```python
from build123d import *

# Parameters (mm, degrees)
EXTRUDE_1_DEPTH     = 33
CUT_EXTRUDE_1_REACH = 63.465
SKETCH_2_R          = 1.5
CUT_EXTRUDE_2_REACH = 63.952
SKETCH_3_R          = 2


with BuildPart() as part:
    # 草图1 → 凸台-拉伸1 (new body)
    with BuildSketch(Plane(origin=(0, 0, 0), x_dir=(1, 0, 0), z_dir=(0, 1, 0))):
        Polygon((0, 0), (43, 0), (43, 33), (40, 33), (40, 3), (0, 3), align=None)
    extrude(amount=EXTRUDE_1_DEPTH)

    # 草图2 → 切除-拉伸1 (cut, up to next)
    with BuildSketch(Plane.ZY.offset(-40), mode=Mode.PRIVATE) as cut_extrude_1_sk1:
        with Locations((-30, 6.5)):
            Circle(SKETCH_2_R)
    cut_extrude_1_tool1 = extrude(cut_extrude_1_sk1.sketch, amount=-CUT_EXTRUDE_1_REACH, mode=Mode.PRIVATE) & part.part
    # 草图2 → 切除-拉伸1 (cut, up to next)
    with BuildSketch(Plane.ZY.offset(-40), mode=Mode.PRIVATE) as cut_extrude_1_sk2:
        with Locations((-30, 26.5)):
            Circle(SKETCH_2_R)
    cut_extrude_1_tool2 = extrude(cut_extrude_1_sk2.sketch, amount=-CUT_EXTRUDE_1_REACH, mode=Mode.PRIVATE) & part.part
    # 草图2 → 切除-拉伸1 (cut, up to next)
    with BuildSketch(Plane.ZY.offset(-40), mode=Mode.PRIVATE) as cut_extrude_1_sk3:
        with Locations((-10, 6.5)):
            Circle(SKETCH_2_R)
    cut_extrude_1_tool3 = extrude(cut_extrude_1_sk3.sketch, amount=-CUT_EXTRUDE_1_REACH, mode=Mode.PRIVATE) & part.part
    # 草图2 → 切除-拉伸1 (cut, up to next)
    with BuildSketch(Plane.ZY.offset(-40), mode=Mode.PRIVATE) as cut_extrude_1_sk4:
        with Locations((-10, 26.5)):
            Circle(SKETCH_2_R)
    cut_extrude_1_tool4 = extrude(cut_extrude_1_sk4.sketch, amount=-CUT_EXTRUDE_1_REACH, mode=Mode.PRIVATE) & part.part
    add(cut_extrude_1_tool1.solids().sort_by_distance((40, 6.5, -30))[0], mode=Mode.SUBTRACT)
    add(cut_extrude_1_tool2.solids().sort_by_distance((40, 26.5, -30))[0], mode=Mode.SUBTRACT)
    add(cut_extrude_1_tool3.solids().sort_by_distance((40, 6.5, -10))[0], mode=Mode.SUBTRACT)
    add(cut_extrude_1_tool4.solids().sort_by_distance((40, 26.5, -10))[0], mode=Mode.SUBTRACT)

    # 草图3 → 切除-拉伸2 (cut, up to next)
    with BuildSketch(Plane(origin=(0, 0, -3), x_dir=(-1, 0, 0), z_dir=(0, 0, -1)), mode=Mode.PRIVATE) as cut_extrude_2_sk1:
        with Locations((-4, 16.5)):
            Circle(SKETCH_3_R)
    cut_extrude_2_tool1 = extrude(cut_extrude_2_sk1.sketch, amount=-CUT_EXTRUDE_2_REACH, mode=Mode.PRIVATE) & part.part
    # 草图3 → 切除-拉伸2 (cut, up to next)
    with BuildSketch(Plane(origin=(0, 0, -3), x_dir=(-1, 0, 0), z_dir=(0, 0, -1)), mode=Mode.PRIVATE) as cut_extrude_2_sk2:
        with Locations((-30, 16.5)):
            Circle(SKETCH_3_R)
    cut_extrude_2_tool2 = extrude(cut_extrude_2_sk2.sketch, amount=-CUT_EXTRUDE_2_REACH, mode=Mode.PRIVATE) & part.part
    # 草图3 → 切除-拉伸2 (cut, up to next)
    with BuildSketch(Plane(origin=(0, 0, -3), x_dir=(-1, 0, 0), z_dir=(0, 0, -1)), mode=Mode.PRIVATE) as cut_extrude_2_sk3:
        with Locations((-17, 16.5)):
            Circle(SKETCH_3_R)
    cut_extrude_2_tool3 = extrude(cut_extrude_2_sk3.sketch, amount=-CUT_EXTRUDE_2_REACH, mode=Mode.PRIVATE) & part.part
    add(cut_extrude_2_tool1.solids().sort_by_distance((4, 16.5, -3))[0], mode=Mode.SUBTRACT)
    add(cut_extrude_2_tool2.solids().sort_by_distance((30, 16.5, -3))[0], mode=Mode.SUBTRACT)
    add(cut_extrude_2_tool3.solids().sort_by_distance((17, 16.5, -3))[0], mode=Mode.SUBTRACT)


solid = part.part
```
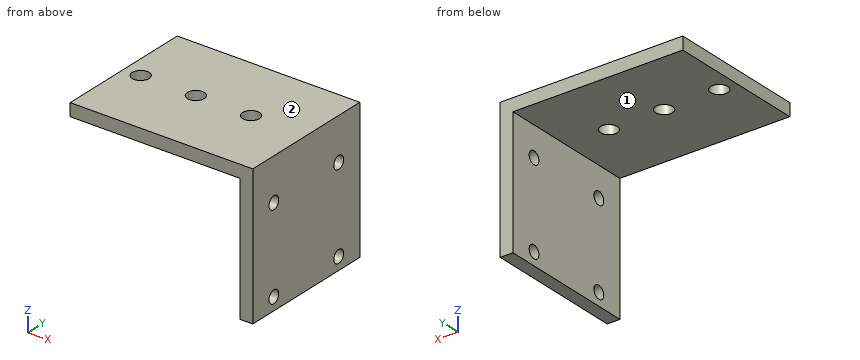
Could you check a few things on this model? Use its own coordinates, in mm. Face numbers are marked on the shaded views. A direction names the side the tool comes from. Round coordinates to 2 decimals unless told otherwise and drop trailing zeros. Loops run counter-clockwise (first coordinate to the right, second up) from the corner with the lowest first, then second, coordinate; pieces in that order, holes last. Notation, with made-up numbers: M 79,55.25 L 122,55.25 A26 ccw 122,82.25 Z; hole C 20.5,89.25 d6. An arc over 180 degrees is marked long. Write item = value, one per line.
1. Will these pins go through, and if not, where does the flat tip stop? P1, Ø12, axis at x = 16, z = -5.5, coming from the -Y side; P2, Ø5, axis at x = 17, y = 16.5, coming from the -Z side; P3, Ø5, axis at y = 6.5, z = -30, coming from the -X side.
Results below:
P1 = 0
P2 = -3
P3 = 40
2. I need wall thicknesses on probe 1 along Y at (x, z) = (42.45, -30); probe 2 along X at (y, z) = (16, -1); probe 3 along Z at (x, y) = (42, 26). Which ranges of each line are inside material? Lowest first, please.
Results below:
probe_1 = 0 to 5, 8 to 25, 28 to 33
probe_2 = 0 to 2.06, 5.94 to 15.06, 18.94 to 28.06, 31.94 to 43
probe_3 = -33 to -31.41, -28.59 to -11.41, -8.59 to 0
3. I want a section at A-A, the plane y = 26.5. Write out the boundary of the cut face in (x, z).
Results below:
outline = M 0,-3 L 40,-3 L 40,-8.5 L 43,-8.5 L 43,0 L 0,0 Z; M 40,-33 L 43,-33 L 43,-31.5 L 40,-31.5 Z; M 40,-28.5 L 43,-28.5 L 43,-11.5 L 40,-11.5 Z
4. I want a section at C-C, the plane y = 16.5. Write out the boundary of the cut face in (x, z), and give its area (3 significant figures).
Results below:
outline = M 0,-3 L 2,-3 L 2,0 L 0,0 Z; M 6,-3 L 15,-3 L 15,0 L 6,0 Z; M 19,-3 L 28,-3 L 28,0 L 19,0 Z; M 32,-3 L 40,-3 L 40,-33 L 43,-33 L 43,0 L 32,0 Z
area = 183 mm²
5. I want a section at D-D, the plane y = 3.5. Write out the boundary of the cut face in (x, z).
Results below:
outline = M 0,-3 L 40,-3 L 40,-33 L 43,-33 L 43,0 L 0,0 Z
6. Which directions (+Z, -Z, +X, -X, +Y, -Y) give clear straight access to the entire face, cutting with the end or side of a thin tool? Please do the marked faces 1 and 2.
Results below:
face_1 = -Z, -X, +Y, -Y
face_2 = +Z, +X, -X, +Y, -Y
7. I want a section at B-B, the plane x = 30. Write out the boundary of the cut face in (y, z).
Results below:
outline = M 0,-3 L 14.5,-3 L 14.5,0 L 0,0 Z; M 18.5,-3 L 33,-3 L 33,0 L 18.5,0 Z
